```python
from build123d import *

# Parameters (mm, degrees)
SKETCH1_R           = 19.25
BOSS_EXTRUDE1_DEPTH = 12
CUT_EXTRUDE1_DEPTH  = 37.292216796
CIRPATTERN1_COUNT   = 20
CUT_EXTRUDE2_DEPTH  = 37.112601679


with BuildPart() as part:
    # Sketch1 → Boss-Extrude1 (new, symmetric)
    with BuildSketch(Plane.XY):
        Circle(SKETCH1_R)
    extrude(amount=BOSS_EXTRUDE1_DEPTH, both=True)

    # Sketch2 → Cut-Extrude1 (cut, through all)
    with BuildSketch(Plane.XY.offset(12)):
        with BuildLine():
            ThreePointArc((0.85, 15.226293049), (0, 15.25), (-0.85, 15.226293049))
            ThreePointArc((-0.85, 15.226293049), (-1.403219848, 17.284232339), (-2.55, 19.080356391))
            ThreePointArc((-2.55, 19.080356391), (0, 19.25), (2.55, 19.080356391))
            ThreePointArc((2.55, 19.080356391), (1.403219848, 17.284232339), (0.85, 15.226293049))
        make_face()
    cut_extrude1 = extrude(amount=-CUT_EXTRUDE1_DEPTH, mode=Mode.SUBTRACT)

    # CirPattern1: Cut-Extrude1 ×20 about axis
    cirpattern1_axis = Axis((0, 0, 0), (0, 0, 1))
    for i in range(1, CIRPATTERN1_COUNT):
        add(cut_extrude1.rotate(cirpattern1_axis, i * 360 / CIRPATTERN1_COUNT), mode=Mode.SUBTRACT)

    # Sketch3 → Cut-Extrude2 (cut, through all)
    with BuildSketch(Plane.XY.offset(12)):
        with BuildLine():
            Line((2, 6.8), (2, 4.582575695))
            ThreePointArc((2, 4.582575695), (0, -5), (-2, 4.582575695))
            Line((-2, 4.582575695), (-2, 6.8))
            Line((-2, 6.8), (2, 6.8))
        make_face()
    extrude(amount=-CUT_EXTRUDE2_DEPTH, mode=Mode.SUBTRACT)


solid = part.part
```
For this review, take the finished solid that the model builds, in its own axes (mm). A direction names the side the tool comes from. Coordinates: 2 decimals unless noted, no trailing zeros. Loops run counter-clockwise (first coordinate to the right, second up) from the corner with the lowest first, then second, coordinate; pieces in that order, holes last. Notation, with made-up numbers: (24.5, -20.75) -> (67.5, -20.75) arc R16 cw to (67.5, -11.75) -> close; hole circle Ø7 at (69.5, 62). An arc over 180 degrees is marked (long way). Return JSON: item names as keys, results as strings. Group by question number.
(1) To check wall thickness, follow L1, parallel to Y at x = -15.5, z = -8; L2, parallel to X at y = 8.5, z = 10.25; L3, parallel to Y at x = 0, z = 0. State the ranges of each line that lie inside material, in increasing order.
(2) Consider section B-B, the plane x = 0. Give the boundary of the cut face in (y, z), plus the area to 3 significant figures.
(3) Consider section A-A, the plane y = 0. Give the boundary of the cut face in (x, z), plus the area to 3 significant figures.
(4) Consider section C-C, the plane x = -16. Give the boundary of the cut face in (y, z).
(5) For pin 1 Ø1.8 at (y, z) = (5.5, -3) entering from +X; pin 2 Ø1.8 at (y, z) = (5.5, -1.5) entering from -X; pin 3 Ø1.5 at (y, z) = (8, -8) entering from +X, all flat-tipped, find the tip position at first contact; note any pin that passes through.
(6) Tool access review of faces 4 (the cylindrical face through (4.01, 16.84, 0.17)), 5 (the cylindrical face through (-6.656, 15.982, 0.168)), 6 (the cylindrical face through (15.25, -0.01, 0.17)), 7 (the cylindrical face through (-13.143, -11.269, 0.168)): name each direction out of +Z, -Z, +X, -X, +Y, -Y from which nothing blocks a thin tool from reaching the whole face with its end or side.
(7) Consider section D-D, the plane y = -6.5. Give the boundary of the cut face in (x, z), plus the area to 3 significant figures.
(8) Mouldability with a two-part tool opening along Y and no side actions: class faces 1 (the cylindrical face through (6.7, 16.03, 0.17)), 2 (the cylindrical face through (-17.257, -1.391, 0.168)), 3 (the cylindrical face through (-1.415, -17.312, 0.168)) as pulls with the +Y half, pulls with the -Y half, needs draft (parallel to the pull), parting line crosses it, or undercut.
Results below:
{
 "1": {"L1": "y = -9.14 to -6.26, -4.01 to -0.89, 0.89 to 4.01, 6.26 to 9.14", "L2": "x = -17.27 to -13.27, -12.66 to 12.66, 13.27 to 17.27", "L3": "y = -15.25 to -5, 6.8 to 15.25"},
 "2": {"outline": "(-15.25, -12) -> (-5, -12) -> (-5, 12) -> (-15.25, 12) -> close; (6.8, -12) -> (15.25, -12) -> (15.25, 12) -> (6.8, 12) -> close", "area": "449 mm2"},
 "3": {"outline": "(-15.25, -12) -> (-5, -12) -> (-5, 12) -> (-15.25, 12) -> close; (5, -12) -> (15.25, -12) -> (15.25, 12) -> (5, 12) -> close", "area": "492 mm2"},
 "4": {"outline": "(-9.18, -12) -> (-6.67, -12) -> (-6.67, 12) -> (-9.18, 12) -> close; (-4.04, -12) -> (-0.98, -12) -> (-0.98, 12) -> (-4.04, 12) -> close; (0.98, -12) -> (4.04, -12) -> (4.04, 12) -> (0.98, 12) -> close; (6.67, -12) -> (9.18, -12) -> (9.18, 12) -> (6.67, 12) -> close"},
 "5": {"pin 1": "stops at x = 15.68", "pin 2": "stops at x = -15.68", "pin 3": "stops at x = 17.36"},
 "6": {"face 4": "+Z, -Z", "face 5": "+Z, -Z, +Y", "face 6": "+Z, -Z, +X", "face 7": "+Z, -Z, -X"},
 "7": {"outline": "(-15.8, -12) -> (15.8, -12) -> (15.8, 12) -> (-15.8, 12) -> close", "area": "758 mm2"},
 "8": {"face 1": "pulls with the +Y half", "face 2": "undercut", "face 3": "pulls with the -Y half"}
}
